from build123d import *

# Parameters (mm, degrees)
F0_W     = 24
F0_H     = 24
F1_DEPTH = 135
F2_W     = 16
F2_H     = 123
F3_DEPTH = 20
F4_R     = 6
F5_DEPTH = 135.001
F6_R     = 4
F7_DEPTH = 25


with BuildPart() as f1:
    # F0 (on Front) → F1 (new body)
    with BuildSketch(Plane.XZ):
        with Locations((12, 12)):
            Rectangle(F0_W, F0_H)
    extrude(amount=F1_DEPTH)

    # F2 (on face) → F3 (cut)
    with BuildSketch(Plane.XY.offset(24)):
        with Locations((12, -67.5)):
            Rectangle(F2_W, F2_H)
    extrude(amount=-F3_DEPTH, mode=Mode.SUBTRACT)

    # F4 (on face) → F5 (cut, through all)
    with BuildSketch(Plane.XZ.offset(135)):
        with Locations((12, 14)):
            Circle(F4_R)
    extrude(amount=-F5_DEPTH, mode=Mode.SUBTRACT)

    # F6 (on face) → F7 (cut)
    with BuildSketch(Plane.XY.offset(4)):
        with Locations((12, -26)):
            Circle(F6_R)
        with Locations((12, -109)):
            Circle(F6_R)
    extrude(amount=-F7_DEPTH, mode=Mode.SUBTRACT)


solid = f1.part
Check sheet for the modelled part. Datum: model origin and axes. Units: mm. A direction names the side the tool comes from. Give positions to 0.01 mm unless a question says otherwise; leave off trailing zeros. Loops run counter-clockwise (first coordinate to the right, second up) from the corner with the lowest first, then second, coordinate; pieces in that order, holes last. Notation, with made-up numbers: M 50,-10.75 L 67,-10.75 A23 cw 67,-2.75 Z; hole C 52,-36.75 d4. An arc over 180 degrees is marked long. Use a Markdown table: item, result. Add a question column.
Q1. Sectioned sample at B-B, the plane y = -26. Record the cut outline in (x, z).
Q2. Tool access check on faces 4 (the cylindrical face through (11.479, -22.034, 2.028)), 5 (the flat face through (20, -68, 14)). Record the directions out of +Z, -Z, +X, -X, +Y, -Y that give a thin tool (end or side, any length) a straight path to the whole face; none if there is none.
Q3. Sectioned sample at D-D, the plane y = -85. Record the cut outline in (x, z), then the cut area to 3 significant figures.
Q4. Mould release check, pull along X, two halves, no side actions. Record for faces 1 (the cylindrical face through (17.54, -132.04, 11.7)), 2 (the flat face through (12, -67, 0)), 3 (the flat face through (0, -67, 12)): pulls with the +X half, pulls with the -X half, needs draft (parallel to the pull), parting line crosses it, or undercut.
Q5. Scan lines: line 1 along Y through (x, z) = (12, 0.9); line 2 along Z through (x, y) = (12, -132.5); line 3 along X through (y, z) = (-122, 14.75). Record each from-to range of solid material in increasing order. Write a range as [from, to].
Q6. Sectioned sample at C-C, the plane z = 14. Record the cut outline in (x, y), then the cut area to 3 significant figures.
Q7. Sectioned sample at A-A, the plane x = 12. Record the cut outline in (y, z).
Verdict:
| question | item | result |
|---|---|---|
| 1 | outline | M 0,0 L 8,0 L 8,4 L 4,4 L 4,24 L 0,24 Z; M 16,0 L 24,0 L 24,24 L 20,24 L 20,4 L 16,4 Z |
| 2 | face 4 | +Z, -Z |
| 2 | face 5 | +Z |
| 3 | outline | M 0,0 L 24,0 L 24,24 L 20,24 L 20,4 L 4,4 L 4,24 L 0,24 Z |
| 3 | area | 256 mm^2 |
| 4 | face 1 | undercut |
| 4 | face 2 | needs draft |
| 4 | face 3 | pulls with the -X half |
| 5 | line 1 | [-135, -113], [-105, -30], [-22, 0] |
| 5 | line 2 | [0, 8], [20, 24] |
| 5 | line 3 | [0, 4], [20, 24] |
| 6 | outline | M 0,-135 L 6,-135 L 6,-129 L 4,-129 L 4,-6 L 6,-6 L 6,0 L 0,0 Z; M 18,-135 L 24,-135 L 24,0 L 18,0 L 18,-6 L 20,-6 L 20,-129 L 18,-129 Z |
| 6 | area | 1,130 mm^2 |
| 7 | outline | M -135,0 L -113,0 L -113,4 L -129,4 L -129,8 L -135,8 Z; M -135,20 L -129,20 L -129,24 L -135,24 Z; M -105,0 L -30,0 L -30,4 L -105,4 Z; M -22,0 L 0,0 L 0,8 L -6,8 L -6,4 L -22,4 Z; M -6,20 L 0,20 L 0,24 L -6,24 Z |
